The listing builds one solid part. Answer for the finished solid, in the listing's coordinates (mm). A direction names the side the tool comes from. Give positions to 0.01 mm unless a question says otherwise; leave off trailing zeros. Order: outer loops, then holes, each group sorted by start corner. A loop starts at its lowest first (then second) coordinate and runs counter-clockwise, first axis right, second up. Notation, with made-up numbers: (79.5, 80.25) -> (127.5, 80.25) arc R3 ccw to (127.5, 84.25) -> close; hole circle Ø4 at (45.5, 73). An arc over 180 degrees is marked (long way). Answer as a JSON object with one key per item and string values. Group by question number.
```python
from build123d import *

# Parameters (mm, degrees)
SKETCH1_R           = 6
BOSS_EXTRUDE1_DEPTH = 20
SKETCH4_R           = 14
BOSS_EXTRUDE2_DEPTH = 10
SKETCH5_R           = 2.25
CUT_EXTRUDE2_DEPTH  = 10
CIRPATTERN1_COUNT   = 6
SKETCH7_R           = 1.75
CUT_EXTRUDE3_DEPTH  = 10
CIRPATTERN2_COUNT   = 3


with BuildPart() as part:
    # Sketch1 → Boss-Extrude1 (new body, symmetric)
    with BuildSketch(Plane(origin=(0, 0, 0), x_dir=(1, 0, 0), z_dir=(0, 1, 0))):
        Circle(SKETCH1_R)
    extrude(amount=BOSS_EXTRUDE1_DEPTH, both=True)

    # Sketch4 → Boss-Extrude2 (add)
    with BuildSketch(Plane(origin=(0, 20, 0), x_dir=(1, 0, 0), z_dir=(0, 1, 0))):
        Circle(SKETCH4_R)
    extrude(amount=BOSS_EXTRUDE2_DEPTH)

    # Sketch5 → Cut-Extrude2 (cut)
    with BuildSketch(Plane(origin=(0, 30, 0), x_dir=(1, 0, 0), z_dir=(0, 1, 0))):
        with Locations((0, 9.5)):
            Circle(SKETCH5_R)
    cut_extrude2 = extrude(amount=-CUT_EXTRUDE2_DEPTH, mode=Mode.SUBTRACT)

    # CirPattern1: Cut-Extrude2 ×6 about axis
    cirpattern1_axis = Axis((0, 0, 0), (0, 1, 0))
    for i in range(1, CIRPATTERN1_COUNT):
        add(cut_extrude2.rotate(cirpattern1_axis, i * 360 / CIRPATTERN1_COUNT), mode=Mode.SUBTRACT)

    # Sketch7 → Cut-Extrude3 (cut)
    with BuildSketch(Plane.XZ.offset(20)):
        with Locations((0, 3)):
            Circle(SKETCH7_R)
    cut_extrude3 = extrude(amount=-CUT_EXTRUDE3_DEPTH, mode=Mode.SUBTRACT)

    # CirPattern2: Cut-Extrude3 ×3 about axis
    cirpattern2_axis = Axis((0, 0, 0), (0, 1, 0))
    for i in range(1, CIRPATTERN2_COUNT):
        add(cut_extrude3.rotate(cirpattern2_axis, i * 360 / CIRPATTERN2_COUNT), mode=Mode.SUBTRACT)


solid = part.part
```
(1) Find the intervals of material crossed by line 1 along Z through (x, y) = (0, 26.5); line 2 along Z through (x, y) = (0, -14.75); line 3 along Y through (x, z) = (1, 2.75), in increasing order. Write a range as [from, to].
(2) Flat-ended cylindrical pins translate along their axes: pin 1 Ø4 at (x, z) = (-8.23, -4.75) entering from +Y; pin 2 Ø8.5 at (x, z) = (-2, 7) entering from -Y; pin 3 Ø1.5 at (y, z) = (20.5, 8.5) entering from -X; pin 4 Ø2 at (y, z) = (15, -2) entering from -X. Find the tip coordinate at first contact, or state that the pin passes through.
(3) A cutting plane is placed at D-D (z = -1.5). Determine the outline of the cut face in (x, y).
(4) Which of the six approach directions +Z, -Z, +X, -X, +Y, -Y give full straight-line access (tool end or side, diameter ignored) to faces 1 (the cylindrical face through (-8.715, 25.07, 6.946)), 2 (the cylindrical face through (0.85, -15.07, -1.42))?
(5) A cutting plane is placed at A-A (x = 0). Determine the outline of the cut face in (y, z).
(6) A cutting plane is placed at C-C (y = 14). Determine the outline of the cut face in (x, z), and give its area (3 significant figures).
(7) A cutting plane is placed at B-B (z = 10.75). Determine the outline of the cut face in (x, y), and give its area (3 significant figures).
(8) For a pull along Z with two mould halves and no side action, classify faces 3 (the cylindrical face through (-0.29, 25.07, -11.73)), 4 (the cylindrical face through (12.932, 24.93, 5.362)), 5 (the flat face through (0, -20, 0)) as +Z half, -Z half, draft (parallel to the pull), parting line (faces both ways), or undercut.
Check sheet entries:
{
 "1": {"line 1": "z = [-14, -11.75], [-7.25, 7.25], [11.75, 14]", "line 2": "z = [-6, 1.25], [4.75, 6]", "line 3": "y = [-10, 30]"},
 "2": {"pin 1": "passes through", "pin 2": "stops at y = -20", "pin 3": "stops at x = -11.66", "pin 4": "stops at x = -5.92"},
 "3": {"outline": "(-13.92, 20) -> (-5.81, 20) -> (-5.81, -20) -> (-4.35, -20) -> (-4.35, -10) -> (-0.85, -10) -> (-0.85, -20) -> (0.85, -20) -> (0.85, -10) -> (4.35, -10) -> (4.35, -20) -> (5.81, -20) -> (5.81, 20) -> (13.92, 20) -> (13.92, 30) -> (-13.92, 30) -> close"},
 "4": {"face 1": "+Y, -Y", "face 2": "-Y"},
 "5": {"outline": "(-20, -6) -> (20, -6) -> (20, -7.25) -> (30, -7.25) -> (30, 7.25) -> (20, 7.25) -> (20, 6) -> (-20, 6) -> (-20, 4.75) -> (-10, 4.75) -> (-10, 1.25) -> (-20, 1.25) -> close; (20, -14) -> (30, -14) -> (30, -11.75) -> (20, -11.75) -> close; (20, 11.75) -> (30, 11.75) -> (30, 14) -> (20, 14) -> close"},
 "6": {"outline": "circle Ø12 at (0, 0)", "area": "113 mm2"},
 "7": {"outline": "(-8.97, 20) -> (-1.87, 20) -> (-1.87, 30) -> (-8.97, 30) -> close; (1.87, 20) -> (8.97, 20) -> (8.97, 30) -> (1.87, 30) -> close", "area": "142 mm2"},
 "8": {"face 3": "undercut", "face 4": "parting line", "face 5": "draft"}
}
